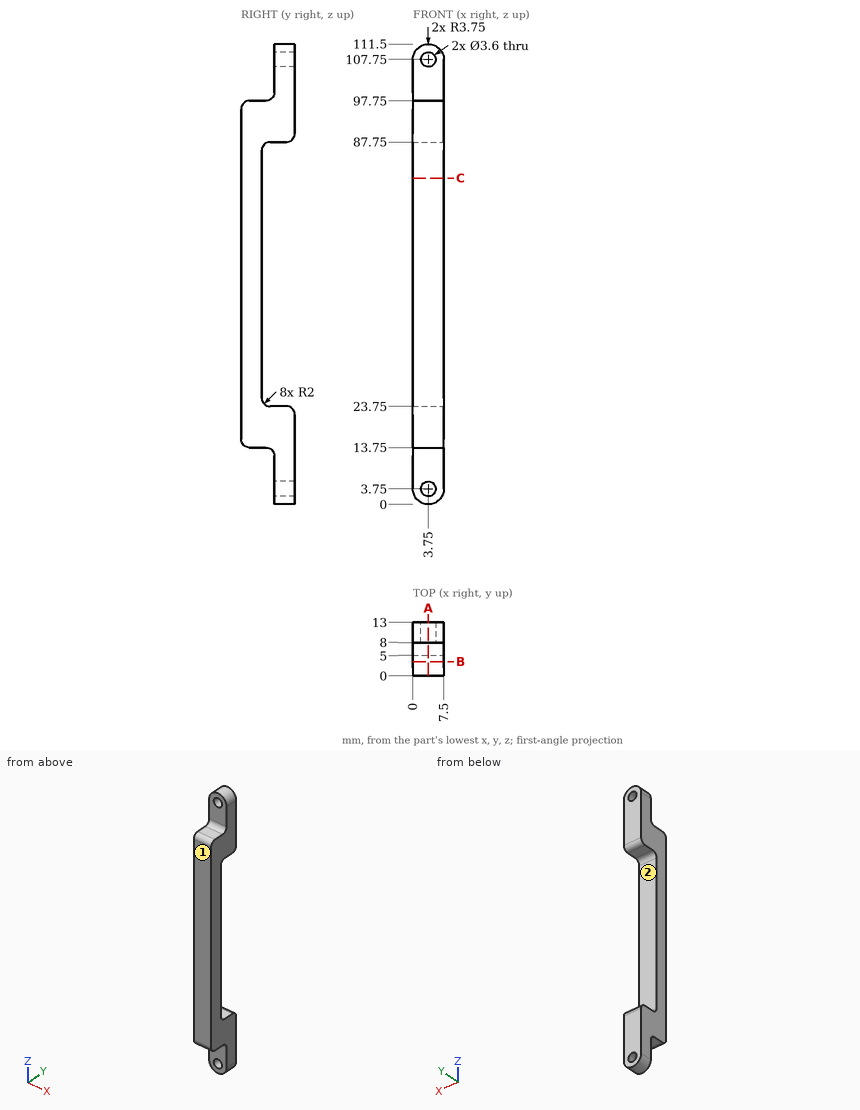
Here's the drawing with two shaded views (mm, measured from the low corner). I have some questions. Give positions to 0.01 mm unless a question says otherwise; leave off trailing zeros. Write each loop counter-clockwise with the first axis right and the second up, starting at its lowest first coordinate (ties: lowest second). Pieces come first, ordered by that corner, then holes. Notation, with made-up numbers: (28, -17.5) -> (51, -17.5) arc R17 cw to (51, -5.5) -> close; hole circle Ø1 at (68.25, -34.75). An arc over 180 degrees is marked (long way). Answer as a JSON object with one key per item and string values. Group by question number.
Item 1: We'd pull the mould along Z, two halves only. Please class the marked faces 1 and 2: +Z half, -Z half, draft (parallel to the pull), parting line (faces both ways), or undercut.
Item 2: I'm going to push flat-ended pins straight in: P1, Ø3, axis at x = 3, y = 4, coming from the -Z side; P2, Ø2, axis at x = 2.5, y = 8.5, coming from the +Z side; P3, Ø6, axis at y = 9, z = 79.5, coming from the +X side; P4, Ø4, axis at x = 5.5, z = 6, coming from the -Y side. Where does each tip first touch, or does it pass through?
Item 3: Please list where these lines run through material, in increasing order: line 1 (Z direction, x = 3.75, y = 10.35); line 2 (Z direction, x = 3.75, y = 11.7); line 3 (X direction, y = 10.8, z = 107.75). Write a range as [from, to].
Item 4: Suppose I cut it at C-C (z = 79). Please give me the cut outline in (x, y), plus the area to 3 significant figures.
Item 5: Suppose I cut it at B-B (y = 3.5). Please give me the cut outline in (x, z).
Item 6: Suppose I cut it at A-A (x = 3.75). Please give me the cut outline in (y, z), plus the area to 4 significant figures.
Findings:
{
 "1": {"face 1": "draft", "face 2": "undercut"},
 "2": {"P1": "stops at z = 13.75", "P2": "stops at z = 111.49", "P3": "passes through", "P4": "stops at y = 8"},
 "3": {"line 1": "z = [0, 1.95], [5.55, 23.75], [87.75, 105.95], [109.55, 111.5]", "line 2": "z = [0, 1.95], [5.55, 23.62], [87.88, 105.95], [109.55, 111.5]", "line 3": "x = [0, 1.95], [5.55, 7.5]"},
 "4": {"outline": "(0, 0) -> (7.5, 0) -> (7.5, 5) -> (0, 5) -> close", "area": "37.5 mm²"},
 "5": {"outline": "(0, 13.75) -> (7.5, 13.75) -> (7.5, 97.75) -> (0, 97.75) -> close"},
 "6": {"outline": "(0, 15.75) arc R2 ccw to (2, 13.75) -> (6, 13.75) arc R2 cw to (8, 11.75) -> (8, 5.55) -> (13, 5.55) -> (13, 21.75) arc R2 ccw to (11, 23.75) -> (7, 23.75) arc R2 cw to (5, 25.75) -> (5, 85.75) arc R2 cw to (7, 87.75) -> (11, 87.75) arc R2 ccw to (13, 89.75) -> (13, 105.95) -> (8, 105.95) -> (8, 99.75) arc R2 cw to (6, 97.75) -> (2, 97.75) arc R2 ccw to (0, 95.75) -> close; (8, 0) -> (13, 0) -> (13, 1.95) -> (8, 1.95) -> close; (8, 109.55) -> (13, 109.55) -> (13, 111.5) -> (8, 111.5) -> close", "area": "681.5 mm²"}
}
